Can you work these out from the model? Positions are in its coordinate system, mm. A direction names the side the tool comes from. Coordinates: 2 decimals unless noted, no trailing zeros. Order: outer loops, then holes, each group sorted by start corner. A loop starts at its lowest first (then second) coordinate and runs counter-clockwise, first axis right, second up. Notation, with made-up numbers: (41.25, -34) -> (96.25, -34) arc R29 cw to (96.25, 0) -> close; hole circle Ø3 at (9.5, -32.5). An arc over 180 degrees is marked (long way). Write item = value, one per line.
```python
from build123d import *

# Parameters (mm, degrees)
BOSS_EXTRU_1_DEPTH      = 20
BOSS_EXTRU_1_DEPTH_BACK = 20
ESQUISSE1_R             = 15
ESQUISSE2_R             = 5
BOSS_EXTRU_2_DEPTH      = 50
BOSS_EXTRU_4_DEPTH      = 5
BOSS_EXTRU_5_START      = 79.35
ESQUISSE5_R             = 5
BOSS_EXTRU_5_DEPTH      = 79.35


with BuildPart() as part:
    # Esquisse1 → Boss.-Extru.1 (new, two sides: drawn at the far end of the back side and taken through both)
    with BuildSketch(Plane.XY.offset(-BOSS_EXTRU_1_DEPTH_BACK)):
        Circle(ESQUISSE1_R)
    extrude(amount=BOSS_EXTRU_1_DEPTH + BOSS_EXTRU_1_DEPTH_BACK)

    # Esquisse2 → Boss.-Extru.2 (add)
    with BuildSketch(Plane.XY.offset(20)):
        Circle(ESQUISSE2_R)
    extrude(amount=BOSS_EXTRU_2_DEPTH)

    # Esquisse3 → Boss.-Extru.4 (add)
    with BuildSketch(Plane.XY.offset(70)):
        Polygon((-1.571578965, 38.361483473), (-5.568168614, 29.787071155), (-12.392312465, 36.338737822), (-15.075770583, 38.915049734), (-15.323219948, 35.203298214), (-15.952493815, 25.76416214), (-24.682553429, 29.408244268), (-28.115474811, 30.841206699), (-27.005375168, 27.290712462), (-24.182346331, 18.261660264), (-33.639278782, 18.506004369), (-37.358028372, 18.602087802), (-35.04030483, 15.69236477), (-29.146238976, 8.292819978), (-38.052833133, 5.104426035), (-41.555173194, 3.85065387), (-38.342847159, 1.974676262), (-30.173770542, -2.796011598), (-37.327141512, -8.98653332), (-40.140061611, -11.420832204), (-36.466975515, -12.009703218), (-27.126167198, -13.507226314), (-31.560212593, -21.863811553), (-33.303812283, -25.149871604), (-29.666036756, -24.37210573), (-20.415024663, -22.39421527), (-21.530902082, -31.788260884), (-21.969698564, -35.482281483), (-18.858535349, -33.442920312), (-10.946719923, -28.256741363), (-8.593723938, -37.419529438), (-7.668455316, -41.022612634), (-5.504084244, -37.997083192), (0, -30.303037958), (5.504084244, -37.997083192), (7.668455316, -41.022612634), (8.593723938, -37.419529438), (10.946719923, -28.256741363), (18.858535349, -33.442920312), (21.969698564, -35.482281483), (21.530902082, -31.788260884), (20.415024663, -22.39421527), (29.666036756, -24.37210573), (33.303812283, -25.149871604), (31.560212593, -21.863811553), (27.126167198, -13.507226314), (36.466975515, -12.009703218), (40.140061611, -11.420832204), (37.327141512, -8.98653332), (30.173770542, -2.796011598), (38.342847159, 1.974676262), (41.555173194, 3.85065387), (38.052833133, 5.104426035), (29.146238976, 8.292819978), (35.04030483, 15.69236477), (37.358028372, 18.602087802), (33.639278782, 18.506004369), (24.182346331, 18.261660264), (27.005375168, 27.290712462), (28.115474811, 30.841206699), (24.682553429, 29.408244268), (15.952493815, 25.76416214), (15.323219948, 35.203298214), (15.075770583, 38.915049734), (12.392312465, 36.338737822), (5.568168614, 29.787071155), (1.571578965, 38.361483473), (0, 41.733199668), align=None)
    extrude(amount=-BOSS_EXTRU_4_DEPTH)

    # Esquisse5 → Boss.-Extru.5 (add)
    with BuildSketch(Plane(origin=(0, 0, -20), x_dir=(-1, 0, 0), z_dir=(0, 0, -1)).offset(BOSS_EXTRU_5_START)):
        Circle(ESQUISSE5_R)
    extrude(amount=-BOSS_EXTRU_5_DEPTH)


solid = part.part
```
Item 1: I want a section at A-A, the plane y = 0. Please give me the cut outline in (x, z), plus the area to 3 significant figures.
A:
outline = (-34.96, 65) -> (-5, 65) -> (-5, 20) -> (-15, 20) -> (-15, -20) -> (-5, -20) -> (-5, -99.35) -> (5, -99.35) -> (5, -20) -> (15, -20) -> (15, 20) -> (5, 20) -> (5, 65) -> (34.96, 65) -> (34.96, 70) -> (-34.96, 70) -> close
area = 2,790 mm2
Item 2: I'm going to push flat-ended pins straight in: P1, Ø1, axis at x = -3.5, y = 26.5, coming from the -Z side; P2, Ø3, axis at x = 0.5, z = -73, coming from the +Y side; P3, Ø1, axis at y = -10.5, z = -3, coming from the +X side. Where does each tip first touch, or does it pass through?
A:
P1 = 65
P2 = 5
P3 = 11.18
Item 3: I want a section at B-B, the plane z = 38. Please give me the cut outline in (x, y), plus the area to 3 significant figures.
A:
outline = circle Ø10 at (0, 0)
area = 78.5 mm2
Item 4: If we mould it in two halves opening along Z, with no side actions, what happens to faces 4 (the cylindrical face through (1.08, -4.88, -60.23)), 5 (the flat face through (0, 0, -99.35)), 6 (the cylindrical face through (-1.08, -4.88, 42.18))? For each: pulls with the +Z half, pulls with the -Z half, needs draft (parallel to the pull), parting line crosses it, or undercut.
A:
face_4 = needs draft
face_5 = pulls with the -Z half
face_6 = undercut
Item 5: For faces 1 (the flat face through (-1, 1, 70)), 2 (the cylindrical face through (-14.985, 0.66, -0.28)), 3 (the flat face through (-4, 4, 20)), which set-ups out of +Z, -Z, +X, -X, +Y, -Y let a thin tool reach every point of the face, with its end or its side?
A:
face_1 = +Z, +X, -X, +Y, -Y
face_2 = -Z
face_3 = none
Item 6: If I drill on probe 1 along Z at (x, y) = (0, 30); probe 2 along X at (y, z) = (-0.5, 53); probe 3 along Y at (x, z) = (4, -11.5), over which ranges is the centre line in solid material (lowest first)?
A:
probe_1 = 65 to 70
probe_2 = -4.97 to 4.97
probe_3 = -14.46 to 14.46
